Geometry: final body of the model. Coordinates: model frame, mm. A direction names the side the tool comes from. Give positions to 0.01 mm unless a question says otherwise; leave off trailing zeros. Write each loop counter-clockwise with the first axis right and the second up, starting at its lowest first coordinate (ties: lowest second). Pieces come first, ordered by that corner, then holes. Notation, with made-up numbers: (29.5, 23.25) -> (87.5, 23.25) arc R27 cw to (87.5, 39.25) -> close; hole circle Ø4 at (47.25, 49). An arc over 180 degrees is marked (long way). Use CSV: the item, a comma, the result in double quotes. Start each with the question number.
1) Section B-B (z = 6.35). Output: boundary loops of the cut face in (x, y) (3 decimals).
2) Section A-A (x = -44.45). Output: boundary loops of the cut face in (y, z) (3 decimals), plus the area to 3 significant figures.
3) Set-up query: faces 1 (the face through (-41.52, -35.47, 7.57)), 2 (the face through (-41, -29.21, 6)), 3 (the face through (41, -29.21, 6)). Return all of +Z, -Z, +X, -X, +Y, -Y with unobstructed straight access to the full face (end or side cutting, diameter ignored); none if empty.
4) Section D-D (z = 1.25). Output: boundary loops of the cut face in (x, y), plus the area to 3 significant figures.
5) Material intervals for line 1 (X direction, y = -34.25, z = 6.35) (3 decimals); line 2 (Z direction, x = 44.45, y = -32.75) (3 decimals); line 3 (Y direction, x = 0.5, z = 7.25), sorted ascending. Write a range as [from, to].
6) Draft query along Z for faces 4 (the face through (41.28, -35.47, 6.21)), 5 (the face through (1, -15, 0)), 6 (the face through (1, -15, 12.7)), 7 (the face through (-50.8, -36, 6)). Return one class per face: pulls with the +Z half, pulls with the -Z half, needs draft (parallel to the pull), parting line crosses it, or undercut.
7) Contact query for flat-ended pins moving along their axis: P1, Ø4, axis at x = -37.5, z = 6, coming from the +Y side; P2, Ø3, axis at x = 13.5, z = 4, coming from the +Y side; P3, Ø4, axis at x = -45.5, z = 8, coming from the +Y side. Output: stop coordinate, or through.
8) Section C-C (y = -38). Output: boundary loops of the cut face in (x, z) (3 decimals).
```python
from build123d import *

# Parameters (mm, degrees)
SKETCH1_R           = 12.7
BOSS_EXTRUDE1_DEPTH = 12.7
SKETCH2_R           = 3.175
CUT_EXTRUDE1_DEPTH  = 13.7
FILLET1_R           = 5.08


with BuildPart() as part:
    # Sketch1 → Boss-Extrude1 (new body)
    with BuildSketch(Plane.XY):
        with BuildLine():
            Line((50.8, -41.91), (-50.8, -41.91))
            Line((-50.8, -41.91), (-50.8, -29.21))
            Line((-50.8, -29.21), (-33.02, -29.21))
            Line((-33.02, -29.21), (-24.716371207, 5.853289191))
            ThreePointArc((-24.716371207, 5.853289191), (0, 25.4), (24.716371207, 5.853289191))
            Line((24.716371207, 5.853289191), (33.02, -29.21))
            Line((33.02, -29.21), (50.8, -29.21))
            Line((50.8, -29.21), (50.8, -41.91))
        make_face()
        Circle(SKETCH1_R, mode=Mode.SUBTRACT)
    extrude(amount=BOSS_EXTRUDE1_DEPTH)

    # Sketch2 → Cut-Extrude1 (cut, through all)
    with BuildSketch(Plane(origin=(0, -29.21, 0), x_dir=(1, 0, 0), z_dir=(0, 1, 0))):
        with Locations((-44.45, -6.35)):
            Circle(SKETCH2_R)
        with Locations((44.45, -6.35)):
            Circle(SKETCH2_R)
    extrude(amount=-CUT_EXTRUDE1_DEPTH, mode=Mode.SUBTRACT)

    # Fillet1
    fillet1_edges = [part.edges().sort_by_distance(p)[0] for p in [
        (-33.02, -29.21, 6.35),
        (33.02, -29.21, 6.35),
    ]]
    fillet(fillet1_edges, radius=FILLET1_R)


solid = part.part
```
Answers follow:
1,outline,"(-50.8, -41.91) -> (-47.625, -41.91) -> (-47.625, -29.21) -> (-50.8, -29.21) -> close; (-41.275, -41.91) -> (41.275, -41.91) -> (41.275, -29.21) -> (37.037, -29.21) arc R5.08 cw to (32.094, -25.301) -> (24.716, 5.853) arc R25.4 ccw to (-24.716, 5.853) -> (-32.094, -25.301) arc R5.08 cw to (-37.037, -29.21) -> (-41.275, -29.21) -> close; (47.625, -41.91) -> (50.8, -41.91) -> (50.8, -29.21) -> (47.625, -29.21) -> close; hole circle Ø25.4 at (0, 0)"
2,outline,"(-41.91, 0) -> (-29.21, 0) -> (-29.21, 3.175) -> (-41.91, 3.175) -> close; (-41.91, 9.525) -> (-29.21, 9.525) -> (-29.21, 12.7) -> (-41.91, 12.7) -> close"
2,area,"80.6 mm^2"
3,face 1,"+Y, -Y"
3,face 2,"+Z, -Z, -X, +Y"
3,face 3,"+Z, -Z, +X, +Y"
4,outline,"(-50.8, -41.91) -> (50.8, -41.91) -> (50.8, -29.21) -> (37.04, -29.21) arc R5.08 cw to (32.09, -25.3) -> (24.72, 5.85) arc R25.4 ccw to (-24.72, 5.85) -> (-32.09, -25.3) arc R5.08 cw to (-37.04, -29.21) -> (-50.8, -29.21) -> close; hole circle Ø25.4 at (0, 0)"
4,area,"3,530 mm^2"
5,line 1,"x = [-50.8, -47.625], [-41.275, 41.275], [47.625, 50.8]"
5,line 2,"z = [0, 3.175], [9.525, 12.7]"
5,line 3,"y = [-41.91, -12.69], [12.69, 25.4]"
6,face 4,"undercut"
6,face 5,"pulls with the -Z half"
6,face 6,"pulls with the +Z half"
6,face 7,"needs draft"
7,P1,"stops at y = -28.97"
7,P2,"stops at y = 22.39"
7,P3,"stops at y = -29.21"
8,outline,"(-50.8, 0) -> (50.8, 0) -> (50.8, 12.7) -> (-50.8, 12.7) -> close; hole circle Ø6.35 at (-44.45, 6.35); hole circle Ø6.35 at (44.45, 6.35)"
